```python
from build123d import *

# Parameters (mm, degrees)
SKETCH2_R           = 1.65
SKETCH2_R_2         = 11
SKETCH2_R_3         = 2.25
BOSS_EXTRUDE1_DEPTH = 3.8


with BuildPart() as part:
    # Sketch2 → Boss-Extrude1 (new body)
    with BuildSketch(Plane.XY):
        with BuildLine():
            Line((-160, 180), (-128, 180))
            ThreePointArc((-128, 180), (-126.585786438, 179.414213562), (-126, 178))
            Line((-126, 178), (-126, 145.072545974))
            Line((-126, 145.072545974), (126, 145.072545974))
            Line((126, 145.072545974), (126, 178))
            ThreePointArc((126, 178), (126.585786438, 179.414213562), (128, 180))
            Line((128, 180), (160, 180))
            Line((160, 180), (160, 55))
            Line((160, 55), (145, 55))
            Line((145, 55), (145, -5))
            Line((145, -5), (160, -5))
            Line((160, -5), (160, -130))
            Line((160, -130), (128, -130))
            ThreePointArc((128, -130), (126.585786438, -129.414213562), (126, -128))
            Line((126, -128), (126, -22))
            ThreePointArc((126, -22), (125.414213562, -20.585786438), (124, -20))
            Line((124, -20), (-124, -20))
            ThreePointArc((-124, -20), (-125.414213562, -20.585786438), (-126, -22))
            Line((-126, -22), (-126, -128))
            ThreePointArc((-126, -128), (-126.585786438, -129.414213562), (-128, -130))
            Line((-128, -130), (-160, -130))
            Line((-160, -130), (-160, -5))
            Line((-160, -5), (-145, -5))
            Line((-145, -5), (-145, 55))
            Line((-145, 55), (-160, 55))
            Line((-160, 55), (-160, 180))
        make_face()
        with Locations(Location((-143.329179578, 122.685954214, 0), (0, 0, 180))):
            Circle(SKETCH2_R, mode=Mode.SUBTRACT)
        with Locations(Location((-143.329179578, 94.016348561, 0), (0, 0, 180))):
            Circle(SKETCH2_R, mode=Mode.SUBTRACT)
        with Locations(Location((143.329179578, 122.685954214, 0), (0, 0, 180))):
            Circle(SKETCH2_R, mode=Mode.SUBTRACT)
        with Locations(Location((143.329179578, 94.016348561, 0), (0, 0, 180))):
            Circle(SKETCH2_R, mode=Mode.SUBTRACT)
        with Locations(Location((143.329179578, 108.351151387, 0), (0, 0, 180))):
            Circle(SKETCH2_R_2, mode=Mode.SUBTRACT)
        with Locations(Location((-143.329179578, 108.351151387, 0), (0, 0, 180))):
            Circle(SKETCH2_R_2, mode=Mode.SUBTRACT)
        with Locations(Location((125.59774802, -0.5, 0), (0, 0, 180))):
            Circle(SKETCH2_R, mode=Mode.SUBTRACT)
        with Locations(Location((125.59774802, 50.5, 0), (0, 0, 180))):
            Circle(SKETCH2_R, mode=Mode.SUBTRACT)
        with Locations(Location((-125.59774802, -0.5, 0), (0, 0, 180))):
            Circle(SKETCH2_R, mode=Mode.SUBTRACT)
        with Locations(Location((-125.59774802, 50.5, 0), (0, 0, 180))):
            Circle(SKETCH2_R, mode=Mode.SUBTRACT)
        with Locations(Location((-29, 10.055, 0), (0, 0, 180))):
            Circle(SKETCH2_R_3, mode=Mode.SUBTRACT)
        with Locations(Location((-29, 39.945, 0), (0, 0, 180))):
            Circle(SKETCH2_R_3, mode=Mode.SUBTRACT)
        with Locations(Location((-53.06, 39.945, 0), (0, 0, 180))):
            Circle(SKETCH2_R_3, mode=Mode.SUBTRACT)
        with Locations(Location((-53.06, 10.055, 0), (0, 0, 180))):
            Circle(SKETCH2_R_3, mode=Mode.SUBTRACT)
        with Locations(Location((53.06, 10.055, 0), (0, 0, 180))):
            Circle(SKETCH2_R_3, mode=Mode.SUBTRACT)
        with Locations(Location((29, 10.055, 0), (0, 0, 180))):
            Circle(SKETCH2_R_3, mode=Mode.SUBTRACT)
        with Locations(Location((29, 39.945, 0), (0, 0, 180))):
            Circle(SKETCH2_R_3, mode=Mode.SUBTRACT)
        with Locations(Location((53.06, 39.945, 0), (0, 0, 180))):
            Circle(SKETCH2_R_3, mode=Mode.SUBTRACT)
        with Locations(Location((143.329179578, -72.685954214, 0), (0, 0, 180))):
            Circle(SKETCH2_R, mode=Mode.SUBTRACT)
        with Locations(Location((143.329179578, -44.016348561, 0), (0, 0, 180))):
            Circle(SKETCH2_R, mode=Mode.SUBTRACT)
        with Locations(Location((143.329179578, -58.351151387, 0), (0, 0, 180))):
            Circle(SKETCH2_R_2, mode=Mode.SUBTRACT)
        with Locations(Location((-143.329179578, -58.351151387, 0), (0, 0, 180))):
            Circle(SKETCH2_R_2, mode=Mode.SUBTRACT)
        with Locations(Location((-143.329179578, -44.016348561, 0), (0, 0, 180))):
            Circle(SKETCH2_R, mode=Mode.SUBTRACT)
        with Locations(Location((-143.329179578, -72.685954214, 0), (0, 0, 180))):
            Circle(SKETCH2_R, mode=Mode.SUBTRACT)
        with Locations(Location((38.179918963, -11.563765186, 0), (0, 0, 180))):
            Circle(SKETCH2_R_3, mode=Mode.SUBTRACT)
        with Locations(Location((-38.179918963, -11.563765186, 0), (0, 0, 180))):
            Circle(SKETCH2_R_3, mode=Mode.SUBTRACT)
        with BuildLine():
            Line((-66, 62.171403079), (-111.59774802, 62.171403079))
            ThreePointArc((-111.59774802, 62.171403079), (-114.426175145, 60.999830204), (-115.59774802, 58.171403079))
            Line((-115.59774802, 58.171403079), (-115.59774802, -8.171403079))
            ThreePointArc((-115.59774802, -8.171403079), (-114.426175145, -10.999830204), (-111.59774802, -12.171403079))
            Line((-111.59774802, -12.171403079), (-66, -12.171403079))
            ThreePointArc((-66, -12.171403079), (-63.171572875, -10.999830204), (-62, -8.171403079))
            Line((-62, -8.171403079), (-62, 58.171403079))
            ThreePointArc((-62, 58.171403079), (-63.171572875, 60.999830204), (-66, 62.171403079))
        make_face(mode=Mode.SUBTRACT)
        with BuildLine():
            Line((66, 62.171403079), (111.59774802, 62.171403079))
            ThreePointArc((111.59774802, 62.171403079), (114.426175145, 60.999830204), (115.59774802, 58.171403079))
            Line((115.59774802, 58.171403079), (115.59774802, -8.171403079))
            ThreePointArc((115.59774802, -8.171403079), (114.426175145, -10.999830204), (111.59774802, -12.171403079))
            Line((111.59774802, -12.171403079), (66, -12.171403079))
            ThreePointArc((66, -12.171403079), (63.171572875, -10.999830204), (62, -8.171403079))
            Line((62, -8.171403079), (62, 58.171403079))
            ThreePointArc((62, 58.171403079), (63.171572875, 60.999830204), (66, 62.171403079))
        make_face(mode=Mode.SUBTRACT)
    extrude(amount=BOSS_EXTRUDE1_DEPTH)


solid = part.part
```
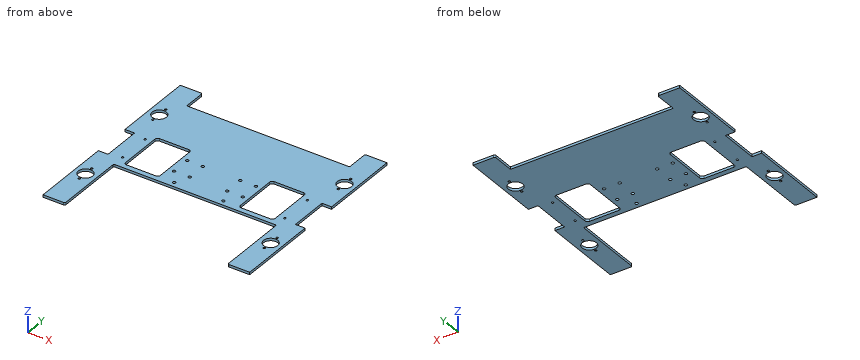
Work out the finished part from the listing and answer in its coordinate system (mm). Coordinates: 2 decimals unless noted, no trailing zeros. Loops run counter-clockwise (first coordinate to the right, second up) from the corner with the lowest first, then second, coordinate; pieces in that order, holes last.
1) Section C-C (x = -18.5) is taken. Give the vertices of the cut face in (y, z).
Results:
outline: (-20, 0) - (145.07, 0) - (145.07, 3.8) - (-20, 3.8) - close
2) Flat-ended cylindrical pins translate along their axes: pin 1 (2 mm diameter, centred on x = -93, z = 1.5, fed in from -Y); pin 2 (1.1 mm diameter, centred on y = 36, z = 1.5, fed in from -X); pin 3 (1.1 mm diameter, centred on x = -77.5, z = 2, fed in from +Y). Find the tip coordinate at first contact, or state that the pin passes through.
Results:
pin 1: stops at y = -20
pin 2: stops at x = -145
pin 3: stops at y = 145.07
3) Consider probe 1 along Y at (x, z) = (-53.06, 0.9) (3 decimals); probe 2 along X at (y, z) = (33, 1.1); probe 3 along X at (y, z) = (94.5, 0.7). Determine where each line is inside the solid, lowest interval first.
Results:
probe 1: y = -20 to 7.805, 12.305 to 37.695, 42.195 to 145.073
probe 2: x = -145 to -115.6, -62 to 62, 115.6 to 145
probe 3: x = -160 to -144.91, -141.75 to 141.75, 144.91 to 160
4) Section A-A (y = -111) is taken. Give the vertices of the cut face in (x, z).
Results:
outline: (-160, 0) - (-126, 0) - (-126, 3.8) - (-160, 3.8) - close; (126, 0) - (160, 0) - (160, 3.8) - (126, 3.8) - close
5) Section B-B (x = -84.5) is taken. Give the vertices of the cut face in (y, z), plus the area to 3 significant figures.
Results:
outline: (-20, 0) - (-12.17, 0) - (-12.17, 3.8) - (-20, 3.8) - close; (62.17, 0) - (145.07, 0) - (145.07, 3.8) - (62.17, 3.8) - close
area: 345 mm2
